```python
from build123d import *

# Parameters (mm, degrees)
SKETCH1_R            = 14
BOSS_EXTRUDE1_DEPTH  = 0.79375
SKETCH2_R            = 2.5
BOSS_EXTRUDE2_DEPTH  = 1.5875
M3_CLEARANCE_HOLE1_D = 3.6
CUT_EXTRUDE1_START   = -10
CUT_EXTRUDE1_DEPTH   = 10


with BuildPart() as part:
    # Sketch1 → Boss-Extrude1 (new, symmetric)
    with BuildSketch(Plane.XY):
        Circle(SKETCH1_R)
    extrude(amount=BOSS_EXTRUDE1_DEPTH, both=True)

    # Sketch2 → Boss-Extrude2 (add, through all)
    with BuildSketch(Plane.XY.offset(0.79375)):
        with BuildLine():
            Line((-13.880322311, 1.826650632), (-22.457257968, -63.347624774))
            ThreePointArc((-22.457257968, -63.347624774), (-21.259114, -67.29682604), (-17.5, -69))
            Line((-17.5, -69), (17.5, -69))
            ThreePointArc((17.5, -69), (21.259114, -67.29682604), (22.457257968, -63.347624774))
            Line((22.457257968, -63.347624774), (13.880322311, 1.826650632))
            Line((13.880322311, 1.826650632), (-13.880322311, 1.826650632))
        make_face()
        with Locations((-10, -61)):
            Circle(SKETCH2_R, mode=Mode.SUBTRACT)
        with Locations((10, -61)):
            Circle(SKETCH2_R, mode=Mode.SUBTRACT)
        with Locations((0, -49)):
            Circle(SKETCH2_R, mode=Mode.SUBTRACT)
    extrude(amount=-BOSS_EXTRUDE2_DEPTH)

    # M3 Clearance Hole1 (through all)
    with Locations(Plane.XY.offset(0.79375)):
        with Locations((5, 8.660254038), (-5, 8.660254038), (-10, 0), (-5, -8.660254038), (5, -8.660254038), (10, 0)):
            Hole(M3_CLEARANCE_HOLE1_D / 2)

    # Sketch5 → Cut-Extrude1 (cut)
    with BuildSketch(Plane(origin=(0, 0, -0.79375), x_dir=(-1, 0, 0), z_dir=(0, 0, -1)).offset(CUT_EXTRUDE1_START)):
        with BuildLine():
            Line((-14.5, -69), (-14.5, -2.882145837))
            Line((-14.5, -2.882145837), (-22.457257968, -63.347624774))
            ThreePointArc((-22.457257968, -63.347624774), (-21.259114, -67.29682604), (-17.5, -69))
            Line((-17.5, -69), (-14.5, -69))
        make_face()
        with BuildLine():
            Line((22.457257968, -63.347624774), (14.5, -2.882145837))
            Line((14.5, -2.882145837), (14.5, -69))
            Line((14.5, -69), (17.5, -69))
            ThreePointArc((17.5, -69), (21.259114, -67.29682604), (22.457257968, -63.347624774))
        make_face()
    extrude(amount=CUT_EXTRUDE1_DEPTH, mode=Mode.SUBTRACT)


solid = part.part
```
Input: part model. Units: mm. Frame: model coordinates. Round coordinates to 2 decimals unless told otherwise and drop trailing zeros. Loops run counter-clockwise (first coordinate to the right, second up) from the corner with the lowest first, then second, coordinate; pieces in that order, holes last. Notation, with made-up numbers: (31, 89.25) - (80, 89.25) arc R20 ccw to (80, 97.25) - close; hole circle Ø2 at (79, 77.5). An arc over 180 degrees is marked (long way). One line per item, written item: value. Start each with the question number.
(1) Ray query, line 1 (Y direction, x = -5, z = 0.35); line 2 (Y direction, x = 10, z = 0); line 3 (Y direction, x = -0.25, z = 0.3). Return the intervals inside material, ascending. Write a range as [from, to].
(2) Draft query along X for faces 1 (the cylindrical face through (-0.54, -51.44, 0.01)), 2 (the flat face through (-14.5, -35, 0)), 3 (the cylindrical face through (0, 14, 0)). Return one class per face: +X half, -X half, draft (parallel to the pull), parting line (faces both ways), or undercut.
(3) Section B-B, the plane y = -49. Return loops of the section in (x, z).
(4) Section C-C, the plane x = 0.5. Return loops of the section in (y, z), plus the area to 3 significant figures.
(5) Section D-D, the plane z = -0.25. Count the separate pieces of the cut face and the enclosed holes in it, plus the area to 3 significant figures.
(6) Section A-A, the plane y = -61. Return loops of the section in (x, z).
(7) Contact query for a flat-ended pin moving along its axis: P1, Ø4, axis at x = 10, y = -61, coming from the -Z side. Output: stop coordinate, or through.
Results below:
1. line 1: [-69, -10.46], [-6.86, 6.86], [10.46, 13.08]
1. line 2: [-69, -63.5], [-58.5, -1.8], [1.8, 9.8]
1. line 3: [-69, -51.49], [-46.51, 14]
2. face 1: undercut
2. face 2: -X half
2. face 3: parting line
3. outline: (-14.5, -0.79) - (-2.5, -0.79) - (-2.5, 0.79) - (-14.5, 0.79) - close; (2.5, -0.79) - (14.5, -0.79) - (14.5, 0.79) - (2.5, 0.79) - close
4. outline: (-69, -0.79) - (-51.45, -0.79) - (-51.45, 0.79) - (-69, 0.79) - close; (-46.55, -0.79) - (13.99, -0.79) - (13.99, 0.79) - (-46.55, 0.79) - close
4. area: 124 mm^2
5. separate pieces: 1
5. enclosed holes: 9
5. area: 2,190 mm^2
6. outline: (-14.5, -0.79) - (-12.5, -0.79) - (-12.5, 0.79) - (-14.5, 0.79) - close; (-7.5, -0.79) - (7.5, -0.79) - (7.5, 0.79) - (-7.5, 0.79) - close; (12.5, -0.79) - (14.5, -0.79) - (14.5, 0.79) - (12.5, 0.79) - close
7. P1: through
